```python
from build123d import *

# Parameters (mm, degrees)
F0_R        = 50
F1_DEPTH    = 100
F2_R        = 4.1
F3_DEPTH    = 20
F4_S5_R     = 4.1
F4_T6_DEPTH = 76


# Not quite as in the source:
# - a fillet or chamfer that OpenCascade refuses, or shapes differently, is made with other operations: its cross-section is extruded or revolved along the edge and cut away or added


with BuildPart() as f1:
    # F0 (on Top) → F1 (new body)
    with BuildSketch(Plane.XY):
        Circle(F0_R)
    extrude(amount=F1_DEPTH)

    # F2 (on face) → F3 (join)
    with BuildSketch(Plane.XY.offset(100)):
        Circle(F2_R)
    extrude(amount=F3_DEPTH)

    # F4: chamfer of 46 on 1 edges, made by hand


with BuildPart() as f4_tool2:
    # F4_s3 → F4_t4 (revolve)
    with BuildSketch(Plane.XZ):
        Polygon((50, 54), (4, 100), (50, 100), align=None)
    revolve(axis=Axis((0, 0, 100), (0, 0, 1)))

    # F4_s5 → F4_t6 (cut, symmetric)
    with BuildSketch(Plane.XY.offset(77)):
        Circle(F4_S5_R)
    extrude(amount=F4_T6_DEPTH, both=True, mode=Mode.SUBTRACT)


with BuildPart() as f1_1:
    add(f1.part)

    # F4_t1: cut F4_tool2
    add(f4_tool2.part, mode=Mode.SUBTRACT)


solid = f1_1.part
```
Source: CAD feature listing. Evaluate the final solid. Frame: model axes, mm. Round coordinates to 2 decimals unless told otherwise and drop trailing zeros. Loops run counter-clockwise (first coordinate to the right, second up) from the corner with the lowest first, then second, coordinate; pieces in that order, holes last.
1. Mould query, pull axis Z, two halves, no side actions, for faces 1 (the cylindrical face through (47.69, 15.02, 26.62)), 2 (the flat face through (-1, 1, 0)), 3 (the flat face through (0, 0, 120)). Classes: released by +Z, released by -Z, zero draft, split by the parting line, or undercut.
2. Section query A-A on x = 0. Output: boundary loops of the cut face in (y, z).
3. Section query C-C on z = 59.5. Output: boundary loops of the cut face in (x, y), and give its area (3 significant figures).
4. Ray query, L1, parallel to Y at x = 20.5, z = 25.5; L2, parallel to Y at x = -11.5, z = 71; L3, parallel to Z at x = -13.5, y = 23.5. Return the intervals inside material, ascending.
5. Section query D-D on z = 23.5. Output: boundary loops of the cut face in (x, y), and give its area (3 significant figures).
6. Contact query for flat-ended pins moving along their axis: pin 1 (5 mm diameter, centred on x = -17.5, y = 29, fed in from +Z); pin 2 (1.5 mm diameter, centred on x = -18, y = -15.5, fed in from -Z); pin 3 (1.5 mm diameter, centred on y = 38, z = 13, fed in from -X); pin 4 (1.5 mm diameter, centred on y = 28, z = 32, fed in from +X). Output: stop coordinate, or through.
Answers below:
1. face 1: zero draft
1. face 2: released by -Z
1. face 3: released by +Z
2. outline: (-50, 0) - (50, 0) - (50, 54) - (4.1, 99.9) - (4.1, 120) - (-4.1, 120) - (-4.1, 99.9) - (-50, 54) - close
3. outline: circle Ø89 at (0, 0)
3. area: 6,220 mm2
4. L1: y = -45.6 to 45.6
4. L2: y = -30.93 to 30.93
4. L3: z = 0 to 76.9
5. outline: circle Ø100 at (0, 0)
5. area: 7,850 mm2
6. pin 1: stops at z = 72.63
6. pin 2: stops at z = 0
6. pin 3: stops at x = -33.35
6. pin 4: stops at x = 41.92
